Verification items for the finished model (mm, model axes). A direction names the side the tool comes from. Give positions to 0.01 mm unless a question says otherwise; leave off trailing zeros. Write each loop counter-clockwise with the first axis right and the second up, starting at its lowest first coordinate (ties: lowest second). Pieces come first, ordered by that corner, then holes.
from build123d import *

# Parameters (mm, degrees)
EXTRUDE_1_DEPTH                  = 10
FILLET_1_R                       = 2
PATTERN_CIRCULAR_2_COUNT         = 3
FILLET_1_OF_PATTERN_CIRCULAR_2_R = 2
CUT_EXTRUDE_START                = -15
SKETCH_3_R                       = 51
CUT_EXTRUDE_1_DEPTH              = 15
SKETCH_4_R                       = 62.618720145
SKETCH_4_R_2                     = 57
CUT_EXTRUDE_2_DEPTH              = 15
CHAMFER_1_SIZE                   = 2
FILLET_2_R                       = 5
SKETCH_5_R                       = 42.5
EXTRUDE_2_DEPTH                  = 3
SKETCH_7_R                       = 39.5
CUT_EXTRUDE_3_DEPTH              = 3
EXTRUDE_START                    = 3
SKETCH_8_W                       = 3
SKETCH_8_H                       = 3
EXTRUDE_4_DEPTH                  = 3


with BuildPart() as part:
    # Эскиз1 → Повернуть1 (revolve)
    with BuildSketch(Plane(origin=(0, 0, 0), x_dir=(1, 0, 0), z_dir=(0, 1, 0))):
        Polygon((0, 0), (-54, 0), (-54, 145), (-51, 145), (-51, 3), (0, 3), align=None)
    revolve(axis=Axis((0, 0, -3), (0, 0, 1)))

    # Эскиз2 → Бобышка-Вытянуть1 (add)
    with BuildSketch(Plane(origin=(57, 0, 0), x_dir=(0, 0, -1), z_dir=(1, 0, 0))):
        Polygon((145, 14), (145, -14), (140, -14), (138.5, 11), (134, 11), (134, 14), align=None)
    extrude_1 = extrude(amount=-EXTRUDE_1_DEPTH)

    # Скругление1
    fillet_1_edges = [part.edges().sort_by_distance(p)[0] for p in [
        (54.576809621, -14, -140),
    ]]
    fillet(fillet_1_edges, radius=FILLET_1_R)

    # Круговой массив2: Бобышка-Вытянуть1 ×3 about axis
    pattern_circular_2_axis = Axis((0, 0, 0), (0, 0, 1))
    for i in range(1, PATTERN_CIRCULAR_2_COUNT):
        add(extrude_1.rotate(pattern_circular_2_axis, i * 360 / PATTERN_CIRCULAR_2_COUNT))

    # Скругление1 of Круговой массив2
    fillet_1_of_pattern_circular_2_edges = [part.edges().sort_by_distance(p)[0] for p in [
        (-15.164049157, 54.264903589, -140),
        (-39.412760463, -40.264903589, -140),
    ]]
    fillet(fillet_1_of_pattern_circular_2_edges, radius=FILLET_1_OF_PATTERN_CIRCULAR_2_R)

    # Эскиз3 → Вырез-Вытянуть1 (cut)
    with BuildSketch(Plane(origin=(0, 0, -145), x_dir=(-1, 0, 0), z_dir=(0, 0, -1)).offset(CUT_EXTRUDE_START)):
        Circle(SKETCH_3_R)
    extrude(amount=CUT_EXTRUDE_1_DEPTH, mode=Mode.SUBTRACT)

    # Эскиз4 → Вырез-Вытянуть2 (cut)
    with BuildSketch(Plane(origin=(0, 0, -145), x_dir=(-1, 0, 0), z_dir=(0, 0, -1))):
        Circle(SKETCH_4_R)
        Circle(SKETCH_4_R_2, mode=Mode.SUBTRACT)
    extrude(amount=-CUT_EXTRUDE_2_DEPTH, mode=Mode.SUBTRACT)

    # Фаска1
    chamfer_1_edges = [part.edges().sort_by_distance(p)[0] for p in [
        (54, 0, 0),
    ]]
    chamfer(chamfer_1_edges, length=CHAMFER_1_SIZE)

    # Скругление2
    fillet_2_edges = [part.edges().sort_by_distance(p)[0] for p in [
        (51, 0, -3),
    ]]
    fillet(fillet_2_edges, radius=FILLET_2_R)

    # Эскиз5 → Бобышка-Вытянуть2 (add)
    with BuildSketch(Plane.XY):
        Circle(SKETCH_5_R)
    extrude(amount=EXTRUDE_2_DEPTH)

    # Эскиз7 → Вырез-Вытянуть3 (cut)
    with BuildSketch(Plane.XY.offset(3)):
        Circle(SKETCH_7_R)
    extrude(amount=-CUT_EXTRUDE_3_DEPTH, mode=Mode.SUBTRACT)

    # Эскиз8 → Бобышка-Вытянуть4 (add)
    with BuildSketch(Plane.XY.offset(EXTRUDE_START)):
        with BuildLine():
            Line((-1.5, -7.858116823), (-1.5, -39.471508712))
            ThreePointArc((-1.5, -39.471508712), (0, -39.5), (1.5, -39.471508712))
            Line((1.5, -39.471508712), (1.5, -7.858116823))
            ThreePointArc((1.5, -7.858116823), (0, -8), (-1.5, -7.858116823))
        make_face()
        with BuildLine():
            ThreePointArc((1.5, 39.471508712), (0, 39.5), (-1.5, 39.471508712))
            Line((-1.5, 39.471508712), (-1.5, 7.858116823))
            ThreePointArc((-1.5, 7.858116823), (0, 8), (1.5, 7.858116823))
            Line((1.5, 7.858116823), (1.5, 39.471508712))
        make_face()
        with BuildLine():
            Line((-1.5, 7.858116823), (-1.5, 1.5))
            Line((-1.5, 1.5), (1.5, 1.5))
            Line((1.5, 1.5), (1.5, 7.858116823))
            ThreePointArc((1.5, 7.858116823), (0, 8), (-1.5, 7.858116823))
        make_face()
        with BuildLine():
            Line((1.5, 7.858116823), (1.5, 1.5))
            Line((1.5, 1.5), (7.858116823, 1.5))
            ThreePointArc((7.858116823, 1.5), (5.656854249, 5.656854249), (1.5, 7.858116823))
        make_face()
        with BuildLine():
            Line((1.5, 1.5), (1.5, -1.5))
            Line((1.5, -1.5), (7.858116823, -1.5))
            ThreePointArc((7.858116823, -1.5), (7.964450219, -0.753347668), (8, 0))
            ThreePointArc((8, 0), (7.964450219, 0.753347668), (7.858116823, 1.5))
            Line((7.858116823, 1.5), (1.5, 1.5))
        make_face()
        with BuildLine():
            ThreePointArc((-39.471508712, 1.5), (-39.5, 0), (-39.471508712, -1.5))
            Line((-39.471508712, -1.5), (-7.858116823, -1.5))
            ThreePointArc((-7.858116823, -1.5), (-8, 0), (-7.858116823, 1.5))
            Line((-7.858116823, 1.5), (-39.471508712, 1.5))
        make_face()
        with BuildLine():
            Line((7.858116823, -1.5), (39.471508712, -1.5))
            ThreePointArc((39.471508712, -1.5), (39.492876536, -0.75013528), (39.5, 0))
            ThreePointArc((39.5, 0), (39.492876536, 0.75013528), (39.471508712, 1.5))
            Line((39.471508712, 1.5), (7.858116823, 1.5))
            ThreePointArc((7.858116823, 1.5), (7.964450219, 0.753347668), (8, 0))
            ThreePointArc((8, 0), (7.964450219, -0.753347668), (7.858116823, -1.5))
        make_face()
        with BuildLine():
            Line((1.5, -1.5), (1.5, -7.858116823))
            ThreePointArc((1.5, -7.858116823), (5.656854249, -5.656854249), (7.858116823, -1.5))
            Line((7.858116823, -1.5), (1.5, -1.5))
        make_face()
        with BuildLine():
            Line((-1.5, -1.5), (-1.5, -7.858116823))
            ThreePointArc((-1.5, -7.858116823), (0, -8), (1.5, -7.858116823))
            Line((1.5, -7.858116823), (1.5, -1.5))
            Line((1.5, -1.5), (-1.5, -1.5))
        make_face()
        Rectangle(SKETCH_8_W, SKETCH_8_H)
        with BuildLine():
            Line((-7.858116823, 1.5), (-1.5, 1.5))
            Line((-1.5, 1.5), (-1.5, 7.858116823))
            ThreePointArc((-1.5, 7.858116823), (-5.656854249, 5.656854249), (-7.858116823, 1.5))
        make_face()
        with BuildLine():
            Line((-7.858116823, -1.5), (-1.5, -1.5))
            Line((-1.5, -1.5), (-1.5, 1.5))
            Line((-1.5, 1.5), (-7.858116823, 1.5))
            ThreePointArc((-7.858116823, 1.5), (-8, 0), (-7.858116823, -1.5))
        make_face()
        with BuildLine():
            ThreePointArc((-7.858116823, -1.5), (-5.656854249, -5.656854249), (-1.5, -7.858116823))
            Line((-1.5, -7.858116823), (-1.5, -1.5))
            Line((-1.5, -1.5), (-7.858116823, -1.5))
        make_face()
    extrude(amount=-EXTRUDE_4_DEPTH)


solid = part.part
Item 1: Depth check by flat-ended pin: pin 1 (4 mm diameter, centred on x = 18.5, z = -109.5, fed in from +Y); pin 2 (10 mm diameter, centred on x = -33.5, z = -59, fed in from +Y); pin 3 (6 mm diameter, centred on y = 22.5, z = -96, fed in from -X). Enter the tip coordinate at first touch or a pass-through.
Answer key:
pin 1: stops at y = 51.42
pin 2: stops at y = 45.87
pin 3: stops at x = -50.36
Item 2: Set-up check for faces 5 (the face through (1, -1, -3)), 6 (the face through (-38, 41, -134)), 7 (the face through (-27.64, 28.22, 1.52)): record each of +Z, -Z, +X, -X, +Y, -Y from which the full face is reachable in a straight line by a thin tool's end or side.
Answer key:
face 5: -Z
face 6: +Z, -X, +Y
face 7: +Z
Item 3: Sectioned sample at A-A on z = -123. Record the cut outline in (x, y), then the cut area to 3 significant figures.
Answer key:
outline: circle Ø108 at (0, 0); hole circle Ø102 at (0, 0)
area: 990 mm2
Item 4: Release check for a two-part mould opening along X. For faces 1 (the face through (5.704, 5.609, 1.521)), 2 (the face through (-33.727, -25.861, 1.479)), 3 (the face through (-28.671, 49.264, -142.021)), 4 (the face through (-16, -53, -134)) record: released by +X, released by -X, zero draft, split by the parting line, or undercut.
Answer key:
face 1: undercut
face 2: split by the parting line
face 3: released by -X
face 4: zero draft
Item 5: Scan lines: line 1 along X through (y, z) = (0, -37); line 2 along Z through (x, y) = (27.5, -8). Record each from-to range of solid material in increasing order.
Answer key:
line 1: x = -54 to -51, 51 to 54
line 2: z = -3 to 0
